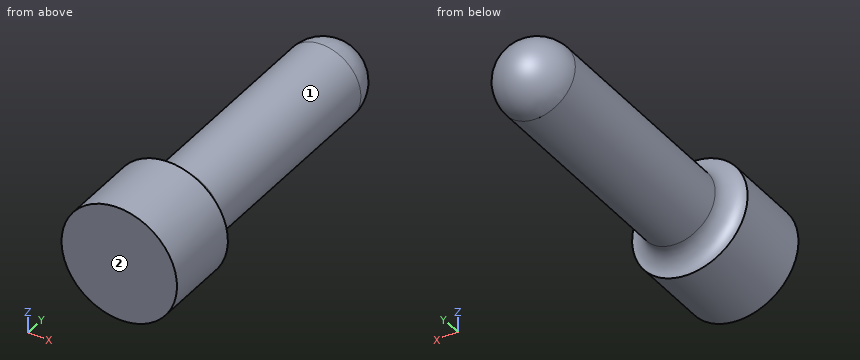
```python
from build123d import *

# Parameters (mm, degrees)
ESBO_O1_R                = 9.9
RESSALTO_EXTRUS_O1_DEPTH = 80
ESBO_O4_R                = 15
RESSALTO_EXTRUS_O2_DEPTH = 20
FILETE3_R                = 5


with BuildPart() as part:
    # Esboço1 → Ressalto-extrusão1 (new body)
    with BuildSketch(Plane(origin=(0, 0, 0), x_dir=(1, 0, 0), z_dir=(0, 1, 0))):
        with Locations(Location((0, 0, 0), (0, 0, 270))):
            Circle(ESBO_O1_R)
    extrude(amount=RESSALTO_EXTRUS_O1_DEPTH)

    # Esboço3 → Revolução1 (revolve)
    with BuildSketch(Plane.XY):
        with BuildLine():
            Line((-9.9, 80), (9.9, 80))
            ThreePointArc((9.9, 80), (0, 89.9), (-9.9, 80))
        make_face()
    revolve(axis=Axis((-9.9, 80, 0), (1, 0, 0)))

    # Esboço4 → Ressalto-extrusão2 (add)
    with BuildSketch(Plane.XZ):
        with Locations(Location((0, 0, 0), (0, 0, 270))):
            Circle(ESBO_O4_R)
    extrude(amount=-RESSALTO_EXTRUS_O2_DEPTH)

    # Filete3
    filete3_edges = [part.edges().sort_by_distance(p)[0] for p in [
        (0, 20, -9.9),
    ]]
    fillet(filete3_edges, radius=FILETE3_R)


solid = part.part
```
Could you check a few things on this model? Use its own coordinates, in mm. Face numbers are marked on the shaded views. A direction names the side the tool comes from. Coordinates: 2 decimals unless noted, no trailing zeros. Order: outer loops, then holes, each group sorted by start corner. A loop starts at its lowest first (then second) coordinate and runs counter-clockwise, first axis right, second up. Notation, with made-up numbers: M -36.75,63.25 L -23.75,63.25 A18 ccw -23.75,85.25 Z; hole C 16.25,-17.5 d7. An arc over 180 degrees is marked long. Use a Markdown table: item, result. Add a question column.
Q1. I want a section at D-D on y = 74. List the corners of the cut face in (x, z) for me, then the cut area to 3 significant figures.
Q2. I'm going to push flat-ended pins straight in: pin 1 (6 mm diameter, centred on y = 65, z = -7, fed in from -X); pin 2 (3 mm diameter, centred on x = 0.5, y = 66.5, fed in from -Z); pin 3 (9 mm diameter, centred on x = -5.5, z = -3, fed in from +Y); pin 4 (1 mm diameter, centred on y = 27, z = 11.5, fed in from -X). Where does each tip first touch, or does it pass through?
Q3. If I drill on L1, parallel to X at y = 55, z = 0.5; L2, parallel to Y at x = -8, z = -8.5; L3, parallel to X at y = 48.5, z = 1.5, over which ranges is the centre line in solid material (lowest first)?
Q4. Which directions (+Z, -Z, +X, -X, +Y, -Y) give clear straight access to the entire face, cutting with the end or side of a thin tool? Please do the marked faces 1 and 2.
Q5. I want a section at C-C on y = 15.5. List the corners of the cut face in (x, z) for me, then the cut area to 3 significant figures.
Q6. I want a section at B-B on x = 0. List the corners of the cut face in (y, z) for me, then the cut area to 3 significant figures.
Q7. I want a section at A-A on z = 0. List the corners of the cut face in (x, y) for me, then the cut area to 3 significant figures.
Checked values:
| question | item | result |
|---|---|---|
| 1 | outline | C 0,0 d19.8 |
| 1 | area | 308 mm² |
| 2 | pin 1 | x = -9.06 |
| 2 | pin 2 | z = -9.9 |
| 2 | pin 3 | y = 89.74 |
| 2 | pin 4 | through |
| 3 | L1 | -9.89 to 9.89 |
| 3 | L2 | 0 to 21.18 |
| 3 | L3 | -9.79 to 9.79 |
| 4 | face 1 | +Y |
| 4 | face 2 | +Z, -Z, +X, -X, -Y |
| 5 | outline | C 0,0 d30 |
| 5 | area | 707 mm² |
| 6 | outline | M 0,-15 L 20,-15 L 20,-14.9 A5 cw 25,-9.9 L 80,-9.9 A9.9 ccw 80,9.9 L 25,9.9 A5 cw 20,14.9 L 20,15 L 0,15 Z |
| 6 | area | 1,950 mm² |
| 7 | outline | M -15,0 L 15,0 L 15,20 L 14.9,20 A5 cw 9.9,25 L 9.9,80 A9.9 ccw -9.9,80 L -9.9,25 A5 cw -14.9,20 L -15,20 Z |
| 7 | area | 1,950 mm² |
